For this review, take the finished solid that the model builds, in its own axes (mm). Give positions to 0.01 mm unless a question says otherwise; leave off trailing zeros. Loops run counter-clockwise (first coordinate to the right, second up) from the corner with the lowest first, then second, coordinate; pieces in that order, holes last. Notation, with made-up numbers: (-8.75, -29) - (33.25, -29) arc R21 ccw to (33.25, -13) - close; hole circle Ø7 at (-38.5, 10). An arc over 180 degrees is marked (long way). Answer in a Markdown table with one row per item.
```python
from build123d import *

# Parameters (mm, degrees)
EXTRUIR1_DEPTH        = 2.5
CROQUIS3_R            = 2.95
CORTAR_EXTRUIR1_DEPTH = 10
CROQUIS4_R            = 2.95
CORTAR_EXTRUIR2_DEPTH = 10


with BuildPart() as part:
    # Croquis2 → Extruir1 (new, symmetric)
    with BuildSketch(Plane.XY):
        with BuildLine():
            Line((100.628572724, -18.418297608), (-100.628572724, -18.418297608))
            ThreePointArc((-100.628572724, -18.418297608), (-119.997393731, 1.886143297), (-100, 21.57181808))
            Line((-100, 21.57181808), (100, 21.57181808))
            ThreePointArc((100, 21.57181808), (119.997393731, 1.886143297), (100.628572724, -18.418297608))
        make_face()
    extrude(amount=EXTRUIR1_DEPTH, both=True)

    # Croquis3 → Cortar-Extruir1 (cut)
    with BuildSketch(Plane.XY.offset(2.5)):
        with Locations(Location((99.999863892, 1.57181808, 0), (0, 0, 180))):
            Circle(CROQUIS3_R)
        with Locations((-99.999863892, 1.57181808)):
            Circle(CROQUIS3_R)
    extrude(amount=-CORTAR_EXTRUIR1_DEPTH, mode=Mode.SUBTRACT)

    # Croquis4 → Cortar-Extruir2 (cut)
    with BuildSketch(Plane.XY.offset(2.5)):
        with Locations((-35, 10)):
            Circle(CROQUIS4_R)
        with Locations(Location((-35, -10, 0), (0, 0, 180))):
            Circle(CROQUIS4_R)
        with Locations((35, -10)):
            Circle(CROQUIS4_R)
        with Locations(Location((35, 10, 0), (0, 0, 180))):
            Circle(CROQUIS4_R)
    extrude(amount=-CORTAR_EXTRUIR2_DEPTH, mode=Mode.SUBTRACT)


solid = part.part
```
1. We need section A-A, the plane x = 35. Give the boundary of the cut face in (y, z), and give its area (3 significant figures).
Values:
| item | result |
|---|---|
| outline | (-18.42, -2.5) - (-12.95, -2.5) - (-12.95, 2.5) - (-18.42, 2.5) - close; (-7.05, -2.5) - (7.05, -2.5) - (7.05, 2.5) - (-7.05, 2.5) - close; (12.95, -2.5) - (21.57, -2.5) - (21.57, 2.5) - (12.95, 2.5) - close |
| area | 141 mm^2 |
2. Clearance check with flat-ended pins moving along their axes: pin 1 (5.5 mm diameter, centred on x = -100, y = 1.57, fed in from +Z); pin 2 (7 mm diameter, centred on x = 35, y = -10, fed in from +Z); pin 3 (2 mm diameter, centred on y = -8.5, z = -1.5, fed in from -X). State where each tip first meets the part, or that it passes through.
Values:
| item | result |
|---|---|
| pin 1 | passes through |
| pin 2 | stops at z = 2.5 |
| pin 3 | stops at x = -117.82 |
3. We need section B-B, the plane z = -1.55. Give the boundary of the cut face in (x, y), and give its area (3 significant figures).
Values:
| item | result |
|---|---|
| outline | (-100.63, -18.42) - (100.63, -18.42) arc R20 ccw to (100, 21.57) - (-100, 21.57) arc R20 ccw to start; hole circle Ø5.9 at (-100, 1.57); hole circle Ø5.9 at (-35, -10); hole circle Ø5.9 at (-35, 10); hole circle Ø5.9 at (35, -10); hole circle Ø5.9 at (35, 10); hole circle Ø5.9 at (100, 1.57) |
| area | 9,090 mm^2 |
4. We need section C-C, the plane y = -10. Give the boundary of the cut face in (x, z), and give its area (3 significant figures).
Values:
| item | result |
|---|---|
| outline | (-116.31, -2.5) - (-37.95, -2.5) - (-37.95, 2.5) - (-116.31, 2.5) - close; (-32.05, -2.5) - (32.05, -2.5) - (32.05, 2.5) - (-32.05, 2.5) - close; (37.95, -2.5) - (116.31, -2.5) - (116.31, 2.5) - (37.95, 2.5) - close |
| area | 1,100 mm^2 |
5. Mouldability with a two-part tool opening along Y and no side actions: class faces 1 (the face through (33.414, 7.513, 0.035)), 2 (the face through (2, 2, 2.5)), 3 (the face through (-1, 21.572, 0)) as released by +Y, released by -Y, zero draft, split by the parting line, or undercut.
Values:
| item | result |
|---|---|
| face 1 | undercut |
| face 2 | zero draft |
| face 3 | released by +Y |
6. Wall thickness on line 1 (Y direction, x = -35, z = -1.15); line 2 (X direction, y = -9, z = -1); line 3 (X direction, y = 2, z = -1.95): over which ranges is each line inside the solid? List them lowest first. Write a range as [from, to].
Values:
| item | result |
|---|---|
| line 1 | y = [-18.42, -12.95], [-7.05, 7.05], [12.95, 21.57] |
| line 2 | x = [-116.98, -37.78], [-32.22, 32.22], [37.78, 116.98] |
| line 3 | x = [-120, -102.92], [-97.08, 97.08], [102.92, 120] |
